from build123d import *

# Parameters (mm, degrees)
F0_W     = 112
F0_H     = 51
F1_DEPTH = 57
F3_DEPTH = 19
F4_DEPTH = 16
F2_W     = 36
F2_H     = 18.5
F5_DEPTH = 56
F6_R     = 8
F7_DEPTH = 16


with BuildPart() as f1:
    # F0 (on Front) → F1 (new body)
    with BuildSketch(Plane.XZ):
        with Locations((56, 25.5)):
            Rectangle(F0_W, F0_H)
    extrude(amount=F1_DEPTH)

    # F2 (on face) → F3 (cut)
    with BuildSketch(Plane.XZ.offset(57)):
        Polygon((93, 51), (19, 51), (19, 32.5), (38, 32.5), (74, 32.5), (93, 32.5), align=None)
    extrude(amount=-F3_DEPTH, mode=Mode.SUBTRACT)

    # F2 (on face) → F4 (join)
    with BuildSketch(Plane.XZ.offset(57)):
        Polygon((19, 32.5), (19, 51), (0, 51), (0, 0), (112, 0), (112, 51), (93, 51), (93, 32.5), (93, 14), (74, 14), (38, 14), (19, 14), align=None)
    extrude(amount=F4_DEPTH)

    # F2 (on face) → F5 (cut)
    with BuildSketch(Plane.XZ.offset(57)):
        with Locations((56, 23.25)):
            Rectangle(F2_W, F2_H)
    extrude(amount=-F5_DEPTH, mode=Mode.SUBTRACT)

    # F6 (on face) → F7 (cut)
    with BuildSketch(Plane(origin=(0, 0, 0), x_dir=(1, 0, 0), z_dir=(0, 0, -1))):
        with Locations((56, 63.874215)):
            Circle(F6_R)
    extrude(amount=-F7_DEPTH, mode=Mode.SUBTRACT)


solid = f1.part
Could you check a few things on this model? Use its own coordinates, in mm. A direction names the side the tool comes from. Round coordinates to 2 decimals unless told otherwise and drop trailing zeros. Write each loop counter-clockwise with the first axis right and the second up, starting at its lowest first coordinate (ties: lowest second). Pieces come first, ordered by that corner, then holes. Notation, with made-up numbers: (68.5, 22) - (104.5, 22) arc R14 cw to (104.5, 41) - close; hole circle Ø5 at (-4, 19.25). An arc over 180 degrees is marked (long way). Put each result on its own line as item: value. Start each with the question number.
(1) I want a section at C-C, the plane z = 43. Please give me the cut outline in (x, y).
(2) Will these pins go through, and if not, where does the flat tip stop? pin 1 (10 mm diameter, centred on x = 55, z = 32.5, fed in from -Y); pin 2 (5.5 mm diameter, centred on x = 50, z = 26.5, fed in from -Y); pin 3 (9.5 mm diameter, centred on x = 80, y = -46.5, fed in from +Z).
(3) I need wall thicknesses on probe 1 along X at (y, z) = (-66, 39); probe 2 along Y at (x, z) = (56, 8.25); probe 3 along Z at (x, y) = (65.5, -26.5). Which ranges of each line are inside material? Lowest first, please.
(4) I want a section at D-D, the plane y = -48.5. Please give me the cut outline in (x, z).
(5) For faces 1 (the flat face through (28, -57, 23)), 2 (the flat face through (38, -29, 23)), 3 (the flat face through (0, -36, 26)), which set-ups out of +Z, -Z, +X, -X, +Y, -Y let a thin tool reach every point of the face, with its end or its side?
(6) I want a section at A-A, the plane y = -35. Please give me the cut outline in (x, z).
(7) Thinking about a two-plate mould opening in X: for faces 4 (the flat face through (55, -36, 0)), 5 (the flat face through (57, -36, 14)), 6 (the flat face through (112, -36, 25)), which applies, released by +X, released by -X, zero draft, split by the parting line, or undercut?
(8) I want a section at B-B, the plane x = 56. Please give me the cut outline in (y, z).
Here are the results:
1. outline: (0, -73) - (19, -73) - (19, -38) - (93, -38) - (93, -73) - (112, -73) - (112, 0) - (0, 0) - close
2. pin 1: stops at y = -38
2. pin 2: stops at y = -1
2. pin 3: stops at z = 32.5
3. probe 1: x = 0 to 19, 93 to 112
3. probe 2: y = -73 to -71.87, -55.87 to 0
3. probe 3: z = 0 to 14, 32.5 to 51
4. outline: (0, 0) - (112, 0) - (112, 51) - (93, 51) - (93, 32.5) - (74, 32.5) - (74, 14) - (38, 14) - (38, 32.5) - (19, 32.5) - (19, 51) - (0, 51) - close
5. face 1: +Z, -Y
5. face 2: -Y
5. face 3: +Z, -Z, -X, +Y, -Y
6. outline: (0, 0) - (112, 0) - (112, 51) - (0, 51) - close; hole (38, 14) - (74, 14) - (74, 32.5) - (38, 32.5) - close
7. face 4: zero draft
7. face 5: undercut
7. face 6: released by +X
8. outline: (-73, 0) - (-71.87, 0) - (-71.87, 14) - (-73, 14) - close; (-55.87, 0) - (0, 0) - (0, 51) - (-38, 51) - (-38, 32.5) - (-1, 32.5) - (-1, 14) - (-55.87, 14) - close
